```python
from build123d import *

# Parameters (mm, degrees)
FILLET1_R          = 0.75
CUT_EXTRUDE2_DEPTH = 3


with BuildPart() as part:
    # Sketch1 → Revolve1 (revolve)
    with BuildSketch(Plane(origin=(0, 0, 0), x_dir=(0, 0, -1), z_dir=(1, 0, 0))):
        with BuildLine():
            Line((0, 0), (60, 0))
            Line((60, 0), (60, 4.75))
            Line((60, 4.75), (6.25, 4.75))
            Line((6.25, 4.75), (6.25, 8.15))
            ThreePointArc((6.25, 8.15), (1.742375921, 5.135294539), (0, 0))
        make_face()
    revolve(axis=Axis((0, 0, 0), (0, 0, -1)))

    # Fillet1
    fillet1_edges = [part.edges().sort_by_distance(p)[0] for p in [
        (0, -8.15, -6.25),
        (0, -4.75, -60),
    ]]
    fillet(fillet1_edges, radius=FILLET1_R)

    # Sketch3 → Cut-Extrude2 (cut)
    with BuildSketch(Plane.XY):
        with BuildLine():
            Line((1.875, -3.247595264), (1.875, -8.652971254))
            Line((1.875, -8.652971254), (-1.875, -8.652971254))
            Line((-1.875, -8.652971254), (-1.875, -3.247595264))
            ThreePointArc((-1.875, -3.247595264), (-3.75, 0), (-1.875, 3.247595264))
            Line((-1.875, 3.247595264), (-1.875, 8.652971254))
            Line((-1.875, 8.652971254), (1.875, 8.652971254))
            Line((1.875, 8.652971254), (1.875, 3.247595264))
            ThreePointArc((1.875, 3.247595264), (3.75, 0), (1.875, -3.247595264))
        make_face()
    extrude(amount=-CUT_EXTRUDE2_DEPTH, mode=Mode.SUBTRACT)


solid = part.part
```
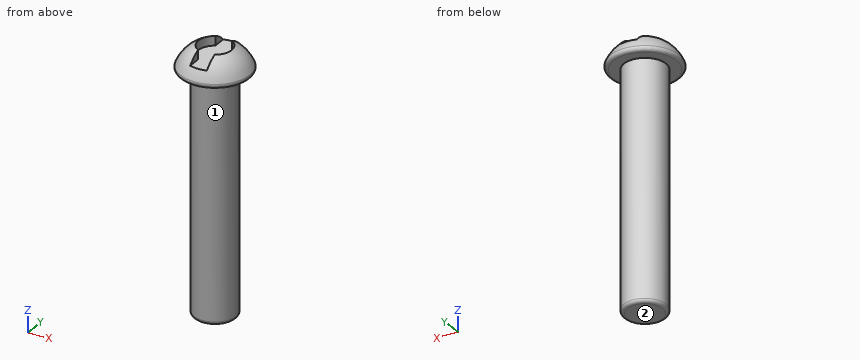
Source: CAD feature listing. Evaluate the final solid. Frame: model axes, mm. Face numbers are marked on the shaded views. A direction names the side the tool comes from. Round coordinates to 2 decimals unless told otherwise and drop trailing zeros. Order: outer loops, then holes, each group sorted by start corner. A loop starts at its lowest first (then second) coordinate and runs counter-clockwise, first axis right, second up. Notation, with made-up numbers: (19, 58) -> (68, 58) arc R16 ccw to (68, 80) -> close; hole circle Ø8 at (7.5, -34). An arc over 180 degrees is marked (long way). Use CSV: the item, a comma, the result in double quotes.
(1) Section A-A on z = -33. Return the cut outline in (x, y).
Report:
outline,"circle Ø9.5 at (0, 0)"
(2) Section B-B on z = -4.5. Return the cut outline in (x, y).
Report:
outline,"circle Ø14.93 at (0, 0)"
(3) Access query for the marked faces 1 and 2. Directions: +Z, -Z, +X, -X, +Y, -Y. A direction counts if a zero-diameter tool reaches every point of the face in a straight line with its end or side. Return the directions, or none.
Report:
face 1,"-Z"
face 2,"-Z, +X, -X, +Y, -Y"
(4) Ray query, L1, parallel to Z at x = -1.5, y = 6; L2, parallel to Z at x = -1, y = -3.5; L3, parallel to X at y = 2.25, z = -46.5. Return the intervals inside material, ascending.
Report:
L1,"-6.25 to -3"
L2,"-60 to -3"
L3,"-4.18 to 4.18"
(5) First-contact query: pin 1 Ø1.1 at (y, z) = (4, -1.5) entering from -X; pin 2 Ø2.5 at (y, z) = (-4.5, -1.5) entering from +X; pin 3 Ø2.5 at (y, z) = (-5, -2) entering from -X. Flat tips, straight axial feed; report the tip coordinate or a pass-through.
Report:
pin 1,"x = -3.95"
pin 2,"x = 4.68"
pin 3,"x = -4.86"
